```python
from build123d import *

# Parameters (mm, degrees)
SKETCH1_R           = 3.96875
BOSS_EXTRUDE2_DEPTH = 5


with BuildPart() as part:
    # Sketch1 → Boss-Extrude2 (new body)
    with BuildSketch(Plane.XY):
        with BuildLine():
            Line((-54.282032303, 22.5), (54.282032303, 22.5))
            ThreePointArc((54.282032303, 22.5), (64.634794107, 21.137033052), (74.282032303, 17.141016151))
            Line((74.282032303, 17.141016151), (85.22114317, 10.825317547))
            ThreePointArc((85.22114317, 10.825317547), (91.47114317, 0), (85.22114317, -10.825317547))
            Line((85.22114317, -10.825317547), (74.282032303, -17.141016151))
            ThreePointArc((74.282032303, -17.141016151), (64.634794107, -21.137033052), (54.282032303, -22.5))
            Line((54.282032303, -22.5), (-54.282032303, -22.5))
            ThreePointArc((-54.282032303, -22.5), (-64.634794107, -21.137033052), (-74.282032303, -17.141016151))
            Line((-74.282032303, -17.141016151), (-85.22114317, -10.825317547))
            ThreePointArc((-85.22114317, -10.825317547), (-91.47114317, 0), (-85.22114317, 10.825317547))
            Line((-85.22114317, 10.825317547), (-74.282032303, 17.141016151))
            ThreePointArc((-74.282032303, 17.141016151), (-64.634794107, 21.137033052), (-54.282032303, 22.5))
        make_face()
        with Locations((-78.97114317, 0)):
            Circle(SKETCH1_R, mode=Mode.SUBTRACT)
        with Locations((78.97114317, 0)):
            Circle(SKETCH1_R, mode=Mode.SUBTRACT)
        Circle(SKETCH1_R, mode=Mode.SUBTRACT)
    extrude(amount=BOSS_EXTRUDE2_DEPTH)


solid = part.part
```
Here's how the part is built. I have some questions about the finished solid (model axes, mm). Coordinates: 2 decimals unless noted, no trailing zeros. Write each loop counter-clockwise with the first axis right and the second up, starting at its lowest first coordinate (ties: lowest second). Pieces come first, ordered by that corner, then holes. Notation, with made-up numbers: M 67.5,68.5 L 107.5,68.5 A21 ccw 107.5,81.5 Z; hole C 26,25.5 d11. An arc over 180 degrees is marked long. Answer as CSV lines item,"result". Start each with the question number.
Q1. Suppose I cut it at C-C, the plane x = 0. List the corners of the cut face in (y, z) for me, then the cut area to 3 significant figures.
Q2. Suppose I cut it at A-A, the plane y = 0. List the corners of the cut face in (x, z) for me, then the cut area to 3 significant figures.
Q3. Suppose I cut it at D-D, the plane y = 13. List the corners of the cut face in (x, z) for me.
Q4. Suppose I cut it at B-B, the plane z = 3.65. List the corners of the cut face in (x, y) for me.
Q5. If we mould it in two halves opening along X, with no side actions, what happens to faces 1 (the flat face through (-79.675, -14.027, 2.465)), 2 (the cylindrical face through (91.47, 0.18, 2.46)), 3 (the cylindrical face through (-82.936, 0.174, 2.465))? For each: pulls with the +X half, pulls with the -X half, needs draft (parallel to the pull), parting line crosses it, or undercut.
Q6. Will these pins go through, and if not, where does the flat tip stop? pin 1 Ø3 at (x, z) = (-61.5, 1) entering from -Y; pin 2 Ø3 at (y, z) = (16, 1.5) entering from +X; pin 3 Ø1.5 at (y, z) = (-9, 0.5) entering from +X.
Q7. I need wall thicknesses on probe 1 along Y at (x, z) = (0, 1.7); probe 2 along X at (y, z) = (-9, 3.4); probe 3 along Y at (x, z) = (-67, 2.85). Which ranges of each line are inside material? Lowest first, please. Write a range as [from, to].
Entries:
1,outline,"M -22.5,0 L -3.97,0 L -3.97,5 L -22.5,5 Z; M 3.97,0 L 22.5,0 L 22.5,5 L 3.97,5 Z"
1,area,"185 mm²"
2,outline,"M -91.47,0 L -82.94,0 L -82.94,5 L -91.47,5 Z; M -75,0 L -3.97,0 L -3.97,5 L -75,5 Z; M 3.97,0 L 75,0 L 75,5 L 3.97,5 Z; M 82.94,0 L 91.47,0 L 91.47,5 L 82.94,5 Z"
2,area,"796 mm²"
3,outline,"M -81.45,0 L 81.45,0 L 81.45,5 L -81.45,5 Z"
4,outline,"M -85.22,-10.83 L -74.28,-17.14 A40 ccw -54.28,-22.5 L 54.28,-22.5 A40 ccw 74.28,-17.14 L 85.22,-10.83 A12.5 ccw 85.22,10.83 L 74.28,17.14 A40 ccw 54.28,22.5 L -54.28,22.5 A40 ccw -74.28,17.14 L -85.22,10.83 A12.5 ccw Z; hole C -78.97,0 d7.94; hole C 0,0 d7.94; hole C 78.97,0 d7.94"
5,face 1,"pulls with the -X half"
5,face 2,"pulls with the +X half"
5,face 3,"undercut"
6,pin 1,"stops at y = -22.09"
6,pin 2,"stops at x = 78.86"
6,pin 3,"stops at x = 88.36"
7,probe 1,"y = [-22.5, -3.97], [3.97, 22.5]"
7,probe 2,"x = [-87.65, 87.65]"
7,probe 3,"y = [-20.42, 20.42]"
